from build123d import *

# Parameters (mm, degrees)
RESSALTO_EXTRUS_O1_DEPTH = 250
CORTE_EXTRUS_O1_DEPTH    = 247
ESBO_O4_W                = 7.5
ESBO_O4_H                = 243
CORTE_EXTRUS_O2_DEPTH    = 245
ESBO_O5_W                = 243
ESBO_O5_H                = 7.5
CORTE_EXTRUS_O3_DEPTH    = 245


with BuildPart() as part:
    # Esboço2 → Ressalto-extrusão1 (new body)
    with BuildSketch(Plane.XY):
        with BuildLine():
            Line((-7.5, 6.160254038), (-7.5, -2.5))
            ThreePointArc((-7.5, -2.5), (-6.035533906, -6.035533906), (-2.5, -7.5))
            Line((-2.5, -7.5), (6.160254038, -7.5))
            ThreePointArc((6.160254038, -7.5), (4.571067812, 4.571067812), (-7.5, 6.160254038))
        make_face()
    extrude(amount=RESSALTO_EXTRUS_O1_DEPTH)

    # Esboço3 → Corte-extrusão1 (cut)
    with BuildSketch(Plane.XY.offset(250)):
        with BuildLine():
            Line((-6.5, 5.562257748), (-6.5, -2.595115556))
            ThreePointArc((-6.5, -2.595115556), (-5.287772695, -5.384664894), (-2.458089295, -6.5))
            Line((-2.458089295, -6.5), (0.796633642, -6.5))
            Line((0.796633642, -6.5), (5.562257748, -6.5))
            ThreePointArc((5.562257748, -6.5), (3.845180245, 3.845180245), (-6.5, 5.562257748))
        make_face()
    extrude(amount=-CORTE_EXTRUS_O1_DEPTH, mode=Mode.SUBTRACT)

    # Esboço4 → Corte-extrusão2 (cut)
    with BuildSketch(Plane.XZ.offset(7.5)):
        with Locations((1.75, 126.5)):
            Rectangle(ESBO_O4_W, ESBO_O4_H)
    extrude(amount=-CORTE_EXTRUS_O2_DEPTH, mode=Mode.SUBTRACT)

    # Esboço5 → Corte-extrusão3 (cut)
    with BuildSketch(Plane.ZY.offset(7.5)):
        with Locations((126.5, 1.75)):
            Rectangle(ESBO_O5_W, ESBO_O5_H)
    extrude(amount=-CORTE_EXTRUS_O3_DEPTH, mode=Mode.SUBTRACT)


solid = part.part
The listing builds one solid part. Answer for the finished solid, in the listing's coordinates (mm). A direction names the side the tool comes from. Coordinates: 2 decimals unless noted, no trailing zeros. Loops run counter-clockwise (first coordinate to the right, second up) from the corner with the lowest first, then second, coordinate; pieces in that order, holes last. Notation, with made-up numbers: M -35.5,42 L -18.5,42 A18 cw -18.5,51 Z; hole C -13,-30.5 d7. An arc over 180 degrees is marked long. Answer in a Markdown table with one row per item.
1) Which of the six approach directions +Z, -Z, +X, -X, +Y, -Y give full straight-line access (tool end or side, diameter ignored) to faces 4 (the flat face through (0, 0, 3)), 5 (the cylindrical face through (-3.189, 7.476, 123.25)), 6 (the flat face through (4, 4, 5))?
Answers below:
| item | result |
|---|---|
| face 4 | +Z |
| face 5 | +Z, -Z |
| face 6 | +X, +Y |
2) Find section B-B (x = 2.25). Determine the outline of the cut face in (y, z), then the cut area to 3 significant figures.
Answers below:
| item | result |
|---|---|
| outline | M -7.5,0 L 6.3,0 L 6.3,5 L 5.11,5 L 5.11,3 L -6.5,3 L -6.5,5 L -7.5,5 Z; M -7.5,248 L -6.5,248 L -6.5,250 L -7.5,250 Z; M 5.11,248 L 6.3,248 L 6.3,250 L 5.11,250 Z |
| area | 50.1 mm^2 |
3) Given pin 1 (6 mm diameter, centred on x = 3.5, z = 67, fed in from +Y); pin 2 (1.1 mm diameter, centred on y = -7, z = 83, fed in from +X); pin 3 (4 mm diameter, centred on x = 1, y = -1, fed in from +Z), each flat-ended and moving along its own axis, determine where each tip first touches the part or whether it passes through.
Answers below:
| item | result |
|---|---|
| pin 1 | y = -2 |
| pin 2 | x = 6.69 |
| pin 3 | z = 3 |
4) Find section C-C (y = 2). Determine the outline of the cut face in (x, z), then the cut area to 3 significant figures.
Answers below:
| item | result |
|---|---|
| outline | M -7.5,0 L 6.43,0 L 6.43,5 L 5.27,5 L 5.27,3 L -6.5,3 L -6.5,5 L -7.5,5 Z; M -7.5,248 L -6.5,248 L -6.5,250 L -7.5,250 Z; M 5.27,248 L 6.43,248 L 6.43,250 L 5.27,250 Z |
| area | 50.5 mm^2 |
5) Find the intervals of material crossed by probe 1 along Z at (x, y) = (2, 6); probe 2 along X at (y, z) = (-2.5, 188.5), in increasing order.
Answers below:
| item | result |
|---|---|
| probe 1 | 0 to 5, 248 to 250 |
| probe 2 | -7.5 to -6.5, 6.48 to 7.5 |
6) Determine the mould class of faces 1 (the flat face through (4, 4, 248)), 2 (the flat face through (-2.3, -6.5, 127.1)), 3 (the cylindrical face through (-6.07, -6, 123.25)) for opening direction X: released by +X, released by -X, zero draft, split by the parting line, or undercut.
Answers below:
| item | result |
|---|---|
| face 1 | zero draft |
| face 2 | undercut |
| face 3 | released by -X |
7) Find section A-A (z = 216). Determine the outline of the cut face in (x, y), then the cut area to 3 significant figures.
Answers below:
| item | result |
|---|---|
| outline | M -7.5,-2.5 A5 ccw -2.5,-7.5 L -2,-7.5 L -2,-6.5 L -2.46,-6.5 A3.97 cw -6.5,-2.6 L -6.5,-2 L -7.5,-2 Z; M -7.5,5.5 L -6.5,5.5 L -6.5,5.56 A9.01 cw -2,6.47 L -2,7.49 A10 ccw -7.5,6.16 Z; M 5.5,-7.5 L 6.16,-7.5 A10 ccw 7.49,-2 L 6.47,-2 A9.01 cw 5.56,-6.5 L 5.5,-6.5 Z |
| area | 19.2 mm^2 |
